```python
from build123d import *

# Parameters (mm, degrees)
BOSS_EXTRUDE1_DEPTH = 1.5
SKETCH3_R           = 2
SKETCH3_R_2         = 2.5
CUT_EXTRUDE1_DEPTH  = 3


with BuildPart() as part:
    # Sketch2 → Boss-Extrude1 (new, symmetric)
    with BuildSketch(Plane(origin=(0, 0, 0), x_dir=(1, 0, 0), z_dir=(0, 1, 0))):
        with BuildLine():
            Line((-41.420454545, -12.342725783), (-41.420454545, 20.380644913))
            ThreePointArc((-41.420454545, 20.380644913), (-39.767396696, 25.250585912), (-35.49137321, 28.107953363))
            Line((-35.49137321, 28.107953363), (28.50862679, 45.259953363))
            ThreePointArc((28.50862679, 45.259953363), (35.449486454, 43.879587063), (38.579545455, 37.532644913))
            Line((38.579545455, 37.532644913), (38.579545455, -29.494725783))
            ThreePointArc((38.579545455, -29.494725783), (35.449486454, -35.841667933), (28.50862679, -37.222034233))
            Line((28.50862679, -37.222034233), (-35.49137321, -20.070034233))
            ThreePointArc((-35.49137321, -20.070034233), (-39.767396696, -17.212666783), (-41.420454545, -12.342725783))
        make_face()
    extrude(amount=BOSS_EXTRUDE1_DEPTH, both=True)

    # Sketch3 → Cut-Extrude1 (cut)
    with BuildSketch(Plane(origin=(0, 1.5, 0), x_dir=(1, 0, 0), z_dir=(0, 1, 0))):
        with Locations(Location((30.579545455, 34.894152552, 0), (0, 0, 270))):
            Circle(SKETCH3_R)
        with Locations(Location((0.579545455, 22.894152552, 0), (0, 0, 270))):
            Circle(SKETCH3_R_2)
        with Locations(Location((-29.420454545, 17.394152552, 0), (0, 0, 270))):
            Circle(SKETCH3_R_2)
        with Locations(Location((30.579545455, -25.105847448, 0), (0, 0, 90))):
            Circle(SKETCH3_R)
        with Locations(Location((0.579545455, -13.105847448, 0), (0, 0, 90))):
            Circle(SKETCH3_R_2)
        with Locations(Location((-29.420454545, -7.605847448, 0), (0, 0, 90))):
            Circle(SKETCH3_R_2)
    extrude(amount=-CUT_EXTRUDE1_DEPTH, mode=Mode.SUBTRACT)


solid = part.part
```
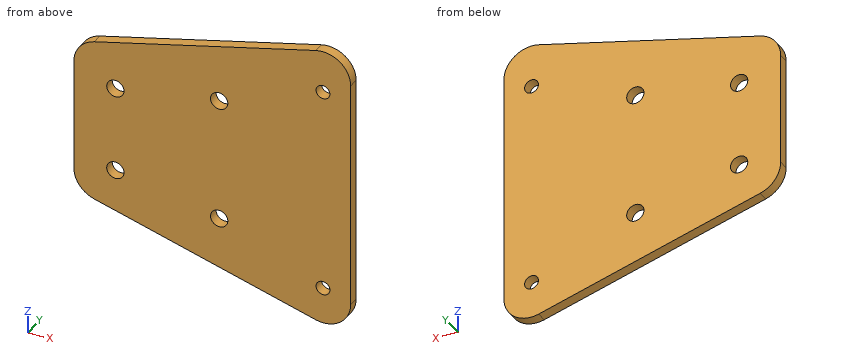
CAD build for the part. Positions are in the model's coordinates, mm. Give positions to 0.01 mm unless a question says otherwise; leave off trailing zeros. Loops run counter-clockwise (first coordinate to the right, second up) from the corner with the lowest first, then second, coordinate; pieces in that order, holes last. Notation, with made-up numbers: (50.5, -26) -> (59.5, -26) arc R24 cw to (59.5, 12) -> close; hole circle Ø1 at (64, 82.5). An arc over 180 degrees is marked (long way). Use a Markdown table: item, result.
1. Slice it at A-A (z = -24). List the corners of the cut face in (x, y), plus the area to 3 significant figures.
Check result:
| item | result |
|---|---|
| outline | (-40.55, -1.5) -> (-1.66, -1.5) -> (-1.66, 1.5) -> (-40.55, 1.5) -> close; (2.82, -1.5) -> (38.58, -1.5) -> (38.58, 1.5) -> (2.82, 1.5) -> close |
| area | 224 mm^2 |
2. Slice it at D-D (z = 6.5). List the corners of the cut face in (x, y).
Check result:
| item | result |
|---|---|
| outline | (-41.42, -1.5) -> (-31.66, -1.5) -> (-31.66, 1.5) -> (-41.42, 1.5) -> close; (-27.18, -1.5) -> (38.58, -1.5) -> (38.58, 1.5) -> (-27.18, 1.5) -> close |
3. Slice it at B-B (y = 0.15). List the corners of the cut face in (x, z).
Check result:
| item | result |
|---|---|
| outline | (-41.42, -20.38) arc R8 ccw to (-35.49, -28.11) -> (28.51, -45.26) arc R8 ccw to (38.58, -37.53) -> (38.58, 29.49) arc R8 ccw to (28.51, 37.22) -> (-35.49, 20.07) arc R8 ccw to (-41.42, 12.34) -> close; hole circle Ø5 at (-29.42, -17.39); hole circle Ø5 at (-29.42, 7.61); hole circle Ø5 at (0.58, -22.89); hole circle Ø5 at (0.58, 13.11); hole circle Ø4 at (30.58, -34.89); hole circle Ø4 at (30.58, 25.11) |
4. Wall check: L1, parallel to Z at x = 30, y = -0.45; L2, parallel to Z at x = 29, y = 0.2; L3, parallel to X at y = 0.45, z = -18. Give the ranges that are in metal, low to high. Write a range as [from, to].
Check result:
| item | result |
|---|---|
| L1 | z = [-45.51, -36.81], [-32.98, 23.19], [27.02, 37.47] |
| L2 | z = [-45.38, -36.12], [-33.67, 23.88], [26.33, 37.34] |
| L3 | x = [-41.42, -31.85], [-26.99, 38.58] |
5. Slice it at C-C (x = -16). List the corners of the cut face in (y, z).
Check result:
| item | result |
|---|---|
| outline | (-1.5, -33.33) -> (1.5, -33.33) -> (1.5, 25.29) -> (-1.5, 25.29) -> close |
